Can you work these out from the model? Positions are in its coordinate system, mm. Face numbers are marked on the shaded views. A direction names the side the tool comes from. Give positions to 0.01 mm unless a question says otherwise; leave off trailing zeros. Loops run counter-clockwise (first coordinate to the right, second up) from the corner with the lowest first, then second, coordinate; pieces in that order, holes last. Notation, with made-up numbers: M -6.5,29.5 L 38.5,29.5 A33 cw 38.5,68.5 Z; hole C 83.5,60.5 d7. An arc over 180 degrees is marked long. Use CSV: the item, a comma, the result in double quotes.
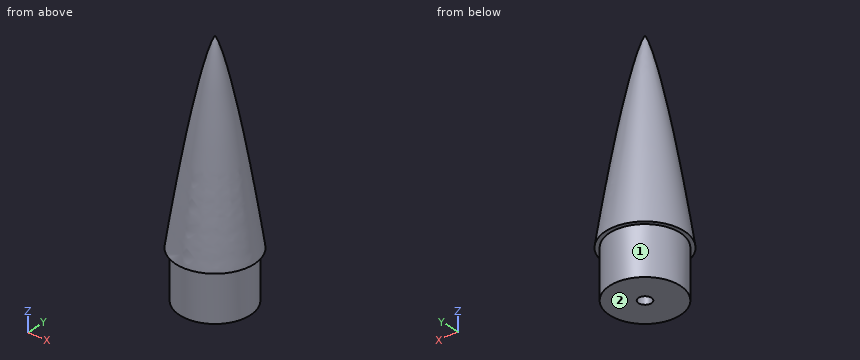
from build123d import *

# Parameters (mm, degrees)
SKETCH2_R                   = 13.992471897
BOSS_EXTRUDE1_DEPTH         = 19.05
F_1_4_20_TAPPED_HOLE1_D     = 5.1054
F_1_4_20_TAPPED_HOLE1_DEPTH = 38.1
F_1_4_20_TAPPED_HOLE1_TIP   = 1.533816902


with BuildPart() as part:
    # Sketch1 → Revolve1 (revolve)
    with BuildSketch(Plane(origin=(0, 0, 0), x_dir=(0, 0, -1), z_dir=(1, 0, 0))):
        with BuildLine():
            Line((76.2, 15.579971897), (76.2, 0))
            Line((76.2, 0), (0, 0))
            add(Edge.make_bspline(
                [(0, 0), (0.002792133, 0.007517657), (0.010102632, 0.021639125), (0.029052268, 0.044540645), (0.058985661, 0.075120576), (0.099333271, 0.110321357), (0.156269016, 0.154766636), (0.239336461, 0.213097121), (0.371995572, 0.296839096), (0.590199779, 0.419955079), (0.965070936, 0.607778944), (1.619855874, 0.897045191), (2.773947, 1.343213722), (4.723814486, 2.000481587), (7.880092454, 2.930618269), (12.115295679, 4.029163257), (17.19406177, 5.217824231), (22.769456129, 6.419578654), (28.368629848, 7.550999177), (33.964865244, 8.624154643), (39.592299094, 9.654907581), (45.189165305, 10.641458188), (50.855832828, 11.604210971), (55.715181086, 12.405681519), (60.047419684, 13.100725468), (63.401347678, 13.631616118), (66.523674112, 14.115542748), (69.466266756, 14.571062691), (73.045302384, 15.109895406), (74.915594162, 15.389572955), (76.2, 15.579971897)],
                knots=[0, 0, 0, 0, 0, 0.000372829, 0.000745658, 0.001374442, 0.002002307, 0.00286818, 0.004118725, 0.006111823, 0.009324733, 0.014564394, 0.023687436, 0.039532586, 0.067072327, 0.110645217, 0.177266519, 0.243887829, 0.310509131, 0.377130436, 0.443751743, 0.510373048, 0.576994355, 0.643615661, 0.710236967, 0.74354762, 0.776858272, 0.810168926, 0.843479579, 0.910100884, 0.910100884, 0.910100884, 0.910100884, 0.910100884], degree=4))
        make_face()
    revolve(axis=Axis((0, 0, -76.2), (0, 0, 1)))

    # Sketch2 → Boss-Extrude1 (add)
    with BuildSketch(Plane(origin=(0, 0, -76.2), x_dir=(-1, 0, 0), z_dir=(0, 0, -1))):
        with Locations(Location((0, 0, 0), (0, 0, 270))):
            Circle(SKETCH2_R)
    extrude(amount=BOSS_EXTRUDE1_DEPTH)

    # 1/4-20 Tapped Hole1
    with Locations(Plane(origin=(0, 0, -95.25), x_dir=(-1, 0, 0), z_dir=(0, 0, -1))):
        with Locations((0, 0)):
            Hole(F_1_4_20_TAPPED_HOLE1_D / 2, depth=F_1_4_20_TAPPED_HOLE1_DEPTH)
            with Locations((0, 0, -(F_1_4_20_TAPPED_HOLE1_DEPTH + F_1_4_20_TAPPED_HOLE1_TIP / 2))):  # 118° drill point
                Cone(0, F_1_4_20_TAPPED_HOLE1_D / 2, F_1_4_20_TAPPED_HOLE1_TIP, mode=Mode.SUBTRACT)


solid = part.part
Q1. For the marked faces 1 and 2, which set-ups out of +Z, -Z, +X, -X, +Y, -Y let a thin tool reach every point of the face, with its end or its side?
Model answer:
face 1,"-Z"
face 2,"-Z, +X, -X, +Y, -Y"
Q2. I want a section at A-A, the plane z = -84. Please give me the cut outline in (x, y).
Model answer:
outline,"C 0,0 d27.98; hole C 0,0 d5.11"
Q3. I'm going to push flat-ended pins straight in: P1, Ø10, axis at x = 0.5, z = -11.5, coming from the -Y side; P2, Ø8, axis at y = 2.5, z = -57.5, coming from the -X side; P3, Ø6, axis at x = 6.5, z = -17, coming from the +Y side; P4, Ø4.5, axis at x = 0, y = 0, coming from the +Z side. Where does each tip first touch, or does it pass through?
Model answer:
P1,"y = -5.04"
P2,"x = -13.25"
P3,"y = 3.93"
P4,"z = 0"
